For this review, take the finished solid that the model builds, in its own axes (mm). Face numbers are marked on the shaded views. A direction names the side the tool comes from. Give positions to 0.01 mm unless a question says otherwise; leave off trailing zeros. Write each loop counter-clockwise with the first axis right and the second up, starting at its lowest first coordinate (ties: lowest second). Pieces come first, ordered by that corner, then holes.
Q1. We need section A-A (y = 20). Write out the cut boundary in (x, z), then the cut area to 3 significant figures.
Q2. For line 1 (Y direction, x = 0, z = -36); line 2 (Y direction, x = 20, z = -37); line 3 (Y direction, x = 0, z = -17.5), list the stretches that pass through material, from the lowest coordinate up.
Q3. We need section D-D (y = 0). Give the number of separate pieces and of enclosed holes in the cut face, then the cut area to 3 significant figures.
Q4. Machinability: for the marked faces 1, 2, 3 and 4, which of the approach directions +Z, -Z, +X, -X, +Y, -Y give a long, thin tool a straight path to every point of the face, cutting with its end or side? Answer none if there is none.
Q5. Insertion check: P1, Ø10, axis at x = 10.5, y = 14, coming from the +Z side; P2, Ø6, axis at x = -7, z = -14, coming from the +Y side; P3, Ø1, axis at x = -8, z = -26, coming from the +Y side. Each pin has a flat end and moves straight along its axis. Give the tip position at first contact, or say it passes through.
Q6. Mouldability with a two-part tool opening along Z and no side actions: class the marked faces 5, 6 and 7 as released by +Z, released by -Z, zero draft, split by the parting line, or undercut.
Q7. We need section C-C (z = -9). Write out the cut boundary in (x, y), then the cut area to 3 significant figures.
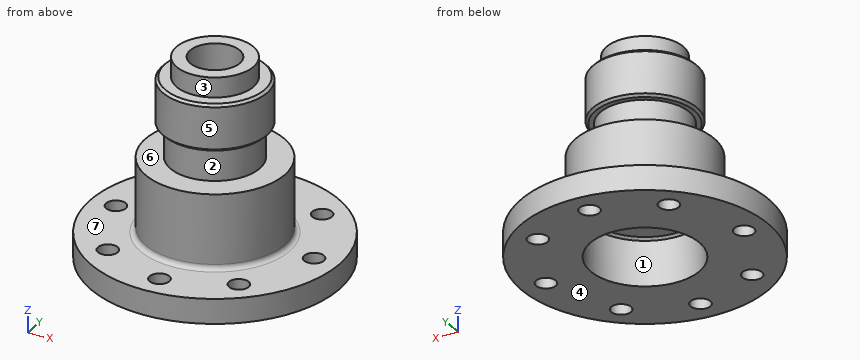
```python
from build123d import *

# Parameters (mm, degrees)
F2_R     = 5
F3_DEPTH = 40
F2_R_2   = 11
F4_DEPTH = 9.6
F2_R_3   = 2
F5_DEPTH = 5
F6_SIZE  = 0.5


with BuildPart() as f1:
    # F0 (on Front) → F1 (revolve)
    with BuildSketch(Plane.XZ):
        with BuildLine():
            Line((7.75, 0), (0, 0))
            Line((0, 0), (0, -40))
            Line((0, -40), (25, -40))
            Line((25, -40), (25, -35))
            Line((25, -35), (15, -35))
            ThreePointArc((15, -35), (14.292893, -34.707107), (14, -34))
            Line((14, -34), (14, -20))
            Line((14, -20), (9, -20))
            Line((9, -20), (9, -13.4))
            Line((9, -13.4), (10.5, -13.4))
            Line((10.5, -13.4), (10.5, -4))
            Line((10.5, -4), (7.75, -4))
            Line((7.75, -4), (7.75, 0))
        make_face()
    revolve(axis=Axis((0, 0, -20), (0, 0, 1)))

    # F2 (on face) → F3 (cut)
    with BuildSketch(Plane(origin=(0, 0, -40), x_dir=(1, 0, 0), z_dir=(0, 0, -1))):
        Circle(F2_R)
    extrude(amount=-F3_DEPTH, mode=Mode.SUBTRACT)

    # F2 (on face) → F4 (cut)
    with BuildSketch(Plane(origin=(0, 0, -40), x_dir=(1, 0, 0), z_dir=(0, 0, -1))):
        Circle(F2_R_2)
        Circle(F2_R, mode=Mode.SUBTRACT)
    extrude(amount=-F4_DEPTH, mode=Mode.SUBTRACT)

    # F2 (on face) → F5 (cut)
    with BuildSketch(Plane(origin=(0, 0, -40), x_dir=(1, 0, 0), z_dir=(0, 0, -1))):
        with Locations((-13.227044, 15.00151)):
            Circle(F2_R_3)
        with Locations((0, 20)):
            Circle(F2_R_3)
        with Locations((13.227044, 15.00151)):
            Circle(F2_R_3)
        with Locations((20, 0)):
            Circle(F2_R_3)
        with Locations((13.227044, -15.00151)):
            Circle(F2_R_3)
        with Locations((0, -20)):
            Circle(F2_R_3)
        with Locations((-13.227044, -15.00151)):
            Circle(F2_R_3)
        with Locations((-20, 0)):
            Circle(F2_R_3)
    extrude(amount=-F5_DEPTH, mode=Mode.SUBTRACT)

    # F6
    f6_edges = [f1.edges().sort_by_distance(p)[0] for p in [
        (-10.5, 0, -13.4),
        (-10.5, 0, -4),
        (-11, 0, -30.4),
    ]]
    chamfer(f6_edges, length=F6_SIZE)


solid = f1.part
```
Computed:
1. outline: (-15, -40) - (-2, -40) - (-2, -35) - (-15, -35) - close; (2, -40) - (15, -40) - (15, -35) - (2, -35) - close
1. area: 130 mm2
2. line 1: y = -25 to -22, -18 to -11, 11 to 18, 22 to 25
2. line 2: y = -15 to -2, 2 to 15
2. line 3: y = -9 to -5, 5 to 9
3. separate pieces: 4
3. enclosed holes: 0
3. area: 493 mm2
4. face 1: -Z
4. face 2: none
4. face 3: +Z
4. face 4: -Z, +X, -X, +Y, -Y
5. P1: stops at z = -20
5. P2: stops at y = 9.62
5. P3: stops at y = 11.82
6. face 5: zero draft
6. face 6: undercut
6. face 7: released by +Z
7. outline: circle Ø21 at (0, 0); hole circle Ø10 at (0, 0)
7. area: 268 mm2
